Geometry: final body of the model. Coordinates: model frame, mm. Round coordinates to 2 decimals unless told otherwise and drop trailing zeros. Loops run counter-clockwise (first coordinate to the right, second up) from the corner with the lowest first, then second, coordinate; pieces in that order, holes last. Notation, with made-up numbers: (26, 16.25) - (48, 16.25) arc R8 ccw to (48, 31.25) - close; hole circle Ø6 at (-25.75, -1). An arc over 180 degrees is marked (long way). Answer in a Markdown table with one row per item. Add a question column.
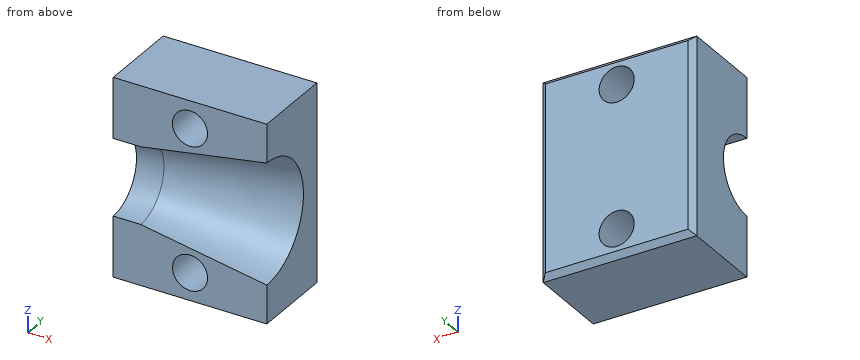
from build123d import *

# Parameters (mm, degrees)
SKETCH_1_W          = 14
SKETCH_1_H          = 18
SKETCH_1_R          = 1.6
EXTRUDE_1_DEPTH     = 4
SKETCH_2_R          = 3.5
CUT_EXTRUDE_1_DEPTH = 2.5
SKETCH_4_R          = 5.5
SKETCH_3_R          = 3.5
CHAMFER_1_SIZE      = 0.5


with BuildPart() as part:
    # 草圖1 → 填料-伸長1 (new body, symmetric)
    with BuildSketch(Plane(origin=(0, 0, 0), x_dir=(1, 0, 0), z_dir=(0, 1, 0))):
        Rectangle(SKETCH_1_W, SKETCH_1_H)
        with Locations((0, 6.5)):
            Circle(SKETCH_1_R, mode=Mode.SUBTRACT)
        with Locations((0, -6.5)):
            Circle(SKETCH_1_R, mode=Mode.SUBTRACT)
    extrude(amount=EXTRUDE_1_DEPTH, both=True)

    # 草圖2 → 除料-伸長1 (cut)
    with BuildSketch(Plane.ZY.offset(7)):
        with Locations((0, -4)):
            Circle(SKETCH_2_R)
    extrude(amount=-CUT_EXTRUDE_1_DEPTH, mode=Mode.SUBTRACT)

    # 草圖4 → 除料-疊層拉伸1 section 0
    with BuildSketch(Plane(origin=(7, 0, 0), x_dir=(0, 0, -1), z_dir=(1, 0, 0))):
        with Locations((0, -4)):
            Circle(SKETCH_4_R)
    # 草圖3 → 除料-疊層拉伸1 section 1
    with BuildSketch(Plane.ZY.offset(4.5)):
        with Locations((0, -4)):
            Circle(SKETCH_3_R)
    loft(mode=Mode.SUBTRACT)

    # 導角1
    chamfer_1_edges = [part.edges().sort_by_distance(p)[0] for p in [
        (-7, 4, 0),
        (0, 4, 9),
        (7, 4, 0),
        (0, 4, -9),
    ]]
    chamfer(chamfer_1_edges, length=CHAMFER_1_SIZE)


solid = part.part
1) Section A-A, the plane z = -6.5. Return the cut outline in (x, y).
2) Section D-D, the plane y = -2.75. Give the number of separate pieces and of enclosed holes in the cut face, and give its area (3 significant figures).
3) Section B-B, the plane y = 3. Return the cut outline in (x, z), and give its area (3 significant figures).
4) Section C-C, the plane x = 0. Return the cut outline in (y, z), and give its area (3 significant figures).
5) Material intervals for line 1 along X through (y, z) = (1.75, -6.5); line 2 along Z through (x, y) = (0, 2.5); line 3 along Z through (x, y) = (0, -1), sorted ascending. Write a range as from..to.
Evaluation:
| question | item | result |
|---|---|---|
| 1 | outline | (-7, -4) - (-1.6, -4) - (-1.6, 4) - (-6.5, 4) - (-7, 3.5) - close; (1.6, -4) - (7, -4) - (7, 3.5) - (6.5, 4) - (1.6, 4) - close |
| 2 | separate pieces | 2 |
| 2 | enclosed holes | 2 |
| 2 | area | 120 mm² |
| 3 | outline | (-7, -9) - (7, -9) - (7, 9) - (-7, 9) - close; hole circle Ø3.2 at (0, -6.5); hole circle Ø3.2 at (0, 6.5) |
| 3 | area | 236 mm² |
| 4 | outline | (-4, -9) - (3.5, -9) - (4, -8.5) - (4, -8.1) - (-4, -8.1) - close; (-4, -4.9) - (4, -4.9) - (4, 4.9) - (-4, 4.9) - (-4, 4.28) arc R4.28 cw to (-4, -4.28) - close; (-4, 8.1) - (4, 8.1) - (4, 8.5) - (3.5, 9) - (-4, 9) - close |
| 4 | area | 63.7 mm² |
| 5 | line 1 | x = -7..-1.6, 1.6..7 |
| 5 | line 2 | z = -9..-8.1, -4.9..4.9, 8.1..9 |
| 5 | line 3 | z = -9..-8.1, -4.9..-3.06, 3.06..4.9, 8.1..9 |
